For this review, take the finished solid that the model builds, in its own axes (mm). A direction names the side the tool comes from. Give positions to 0.01 mm unless a question says otherwise; leave off trailing zeros. Loops run counter-clockwise (first coordinate to the right, second up) from the corner with the lowest first, then second, coordinate; pieces in that order, holes last. Notation, with made-up numbers: (36, 15) -> (73, 15) arc R28 cw to (73, 47) -> close; hole circle Ø10 at (33, -38). An arc over 180 degrees is marked (long way). Write each question's results on one line, items separated by ' | '. Start each with the question number.
```python
from build123d import *

# Parameters (mm, degrees)
BOSS_EXTRUDE1_DEPTH = 609.6
CUT_EXTRUDE1_DEPTH  = 2.794
LPATTERN1_COUNT     = 12
LPATTERN1_PITCH     = 50.8


with BuildPart() as part:
    # Sketch1 → Boss-Extrude1 (new body)
    with BuildSketch(Plane.XY):
        with BuildLine():
            Line((-36.22675, 20.6375), (-3.46075, 20.6375))
            ThreePointArc((-3.46075, 20.6375), (-1.013630207, 19.623869793), (0, 17.17675))
            Line((0, 17.17675), (0, -17.17675))
            ThreePointArc((0, -17.17675), (-1.013630207, -19.623869793), (-3.46075, -20.6375))
            Line((-3.46075, -20.6375), (-36.22675, -20.6375))
            ThreePointArc((-36.22675, -20.6375), (-39.796401808, -19.158901808), (-41.275, -15.58925))
            Line((-41.275, -15.58925), (-41.275, -14.57325))
            ThreePointArc((-41.275, -14.57325), (-40.261369793, -12.126130207), (-37.81425, -11.1125))
            Line((-37.81425, -11.1125), (-35.5346, -11.1125))
            ThreePointArc((-35.5346, -11.1125), (-34.1376, -12.5095), (-35.5346, -13.9065))
            Line((-35.5346, -13.9065), (-37.81425, -13.9065))
            ThreePointArc((-37.81425, -13.9065), (-38.285713446, -14.101786554), (-38.481, -14.57325))
            Line((-38.481, -14.57325), (-38.481, -15.58925))
            ThreePointArc((-38.481, -15.58925), (-37.820745461, -17.183245461), (-36.22675, -17.8435))
            Line((-36.22675, -17.8435), (-3.46075, -17.8435))
            ThreePointArc((-3.46075, -17.8435), (-2.989286554, -17.648213446), (-2.794, -17.17675))
            Line((-2.794, -17.17675), (-2.794, 17.17675))
            ThreePointArc((-2.794, 17.17675), (-2.989286554, 17.648213446), (-3.46075, 17.8435))
            Line((-3.46075, 17.8435), (-36.22675, 17.8435))
            ThreePointArc((-36.22675, 17.8435), (-37.820745461, 17.183245461), (-38.481, 15.58925))
            Line((-38.481, 15.58925), (-38.481, 14.57325))
            ThreePointArc((-38.481, 14.57325), (-38.285713446, 14.101786554), (-37.81425, 13.9065))
            Line((-37.81425, 13.9065), (-35.5346, 13.9065))
            ThreePointArc((-35.5346, 13.9065), (-34.1376, 12.5095), (-35.5346, 11.1125))
            Line((-35.5346, 11.1125), (-37.81425, 11.1125))
            ThreePointArc((-37.81425, 11.1125), (-40.261369793, 12.126130207), (-41.275, 14.57325))
            Line((-41.275, 14.57325), (-41.275, 15.58925))
            ThreePointArc((-41.275, 15.58925), (-39.796401808, 19.158901808), (-36.22675, 20.6375))
        make_face()
    extrude(amount=-BOSS_EXTRUDE1_DEPTH)

    # Sketch2 → Cut-Extrude1 (cut)
    with BuildSketch(Plane(origin=(0, 0, 0), x_dir=(0, 0, -1), z_dir=(1, 0, 0))):
        with BuildLine():
            Line((18.25625, 7.14375), (32.54375, 7.14375))
            ThreePointArc((32.54375, 7.14375), (39.6875, 0), (32.54375, -7.14375))
            Line((32.54375, -7.14375), (18.25625, -7.14375))
            ThreePointArc((18.25625, -7.14375), (11.1125, 0), (18.25625, 7.14375))
        make_face()
    cut_extrude1 = extrude(amount=-CUT_EXTRUDE1_DEPTH, mode=Mode.SUBTRACT)

    # LPattern1: Cut-Extrude1 ×12
    with Locations(*[(0, 0, -i * LPATTERN1_PITCH) for i in range(1, LPATTERN1_COUNT)]):
        add(cut_extrude1, mode=Mode.SUBTRACT)


solid = part.part
```
1. Wall thickness on L1, parallel to Y at x = -28, z = -583; L2, parallel to Y at x = -38, z = -467; L3, parallel to X at y = 15, z = -534.5 (3 decimals): over which ranges is each line inside the solid? List them lowest first.
2. We need section C-C (z = -150.5). Write out the cut boundary in (x, y) (1 decimal), plus the area to 3 significant figures.
3. For pin 1 Ø1.4 at (x, z) = (-1, -225.5) entering from -Y; pin 2 Ø1.4 at (x, z) = (-1, -129) entering from +Y; pin 3 Ø0.8 at (x, z) = (-1, -383) entering from -Y, all flat-tipped, find the tip position at first contact; note any pin that passes through.
4. We need section B-B (y = 0). Count the separate pieces of the cut face and the enclosed holes in it, plus the area to 3 significant figures.
5. Draft analysis for pull direction X (two halves, no side actions). For faces 1 (the flat face through (0, 0, -301)), 2 (the flat face through (-2, 0, -609.6)), 3 (the flat face through (-20, -17.844, -301)), state which applies: released by +X, released by -X, zero draft, split by the parting line, or undercut.
6. We need section A-A (x = -14.5). Write out the cut boundary in (y, z).
7. Machinability: for faces 4 (the flat face through (-20, 20.638, -301)), 5 (the flat face through (-2.794, 0, -301)), which of the approach directions +Z, -Z, +X, -X, +Y, -Y give a long, thin tool a straight path to every point of the face, cutting with its end or side? Answer none if there is none.
Response:
1) L1: y = -20.64 to -17.84, 17.84 to 20.64 | L2: y = -20.32 to -16.98, -13.93 to -11.12, 11.12 to 13.93, 16.98 to 20.32 | L3: x = -41.275 to -38.481, -2.794 to 0
2) outline: (-41.3, -15.6) arc R5 ccw to (-36.2, -20.6) -> (-3.5, -20.6) arc R3.5 ccw to (0, -17.2) -> (0, 17.2) arc R3.5 ccw to (-3.5, 20.6) -> (-36.2, 20.6) arc R5 ccw to (-41.3, 15.6) -> (-41.3, 14.6) arc R3.5 ccw to (-37.8, 11.1) -> (-35.5, 11.1) arc R1.4 ccw to (-35.5, 13.9) -> (-37.8, 13.9) arc R0.7 cw to (-38.5, 14.6) -> (-38.5, 15.6) arc R2.3 cw to (-36.2, 17.8) -> (-3.5, 17.8) arc R0.7 cw to (-2.8, 17.2) -> (-2.8, -17.2) arc R0.7 cw to (-3.5, -17.8) -> (-36.2, -17.8) arc R2.3 cw to (-38.5, -15.6) -> (-38.5, -14.6) arc R0.7 cw to (-37.8, -13.9) -> (-35.5, -13.9) arc R1.4 ccw to (-35.5, -11.1) -> (-37.8, -11.1) arc R3.5 ccw to (-41.3, -14.6) -> close | area: 372 mm2
3) pin 1: stops at y = -20.16 | pin 2: stops at y = 20.16 | pin 3: stops at y = -19.96
4) separate pieces: 13 | enclosed holes: 0 | area: 745 mm2
5) face 1: released by +X | face 2: zero draft | face 3: undercut
6) outline: (-20.64, -609.6) -> (-17.84, -609.6) -> (-17.84, 0) -> (-20.64, 0) -> close; (17.84, -609.6) -> (20.64, -609.6) -> (20.64, 0) -> (17.84, 0) -> close
7) face 4: +Z, -Z, +X, -X, +Y | face 5: +Z, -Z
